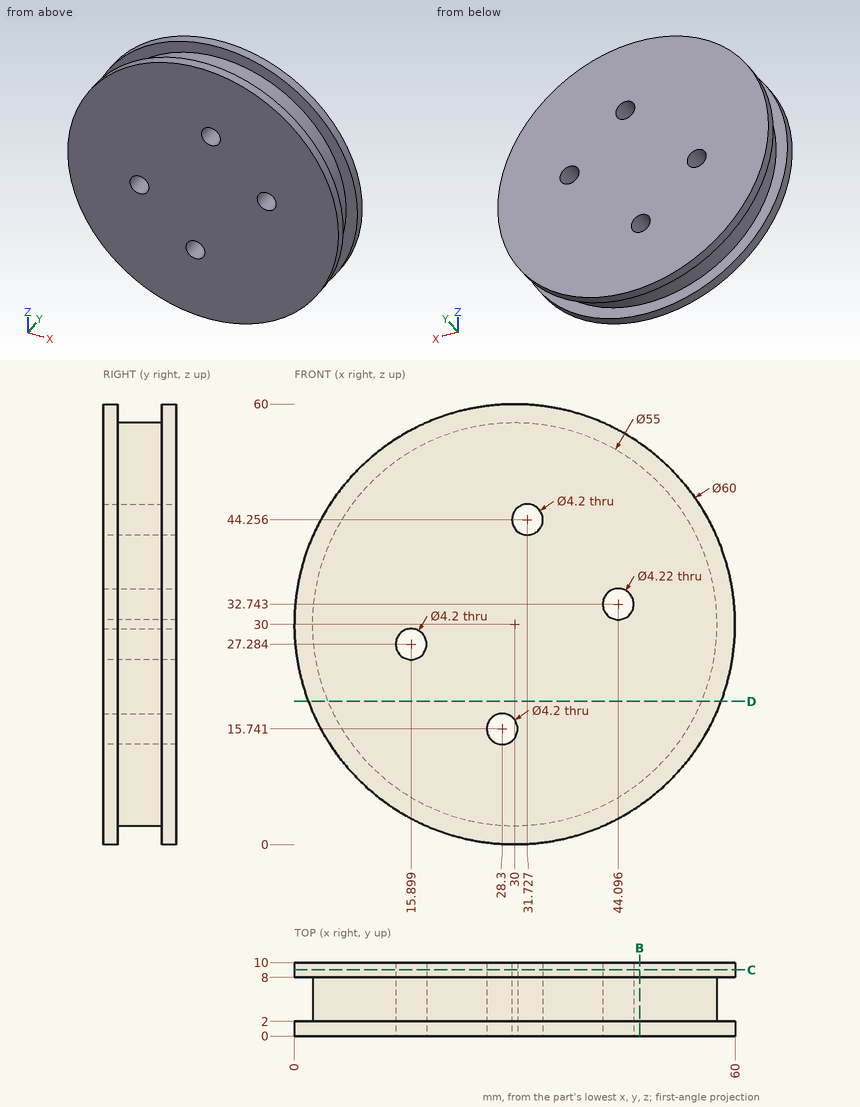
Input: dimensioned drawing with shaded views. Units: mm. Origin: part minimum x, y, z. Coordinates: 2 decimals unless noted, no trailing zeros. Write each loop counter-clockwise with the first axis right and the second up, starting at its lowest first coordinate (ties: lowest second). Pieces come first, ordered by that corner, then holes. Notation, with made-up numbers: M -26,-23 L 29,-23 A13 ccw 29,0 Z; hole C 34,-39.5 d10. An arc over 180 degrees is marked long. Answer as a JSON object with one key per item and string values. Group by question number.
(1) Section D-D on z = 19.5. Output: boundary loops of the cut face in (x, y), plus the area to 3 significant figures.
(2) Ray query, line 1 along Y through (x, z) = (58, 23); line 2 along Z through (x, y) = (32.5, 1.5) (1 decimal); line 3 along X through (y, z) = (5, 43) (1 decimal). Return the intervals inside material, ascending. Write a range as [from, to].
(3) Section B-B on x = 47. Output: boundary loops of the cut face in (y, z) (1 decimal).
(4) Contact query for a flat-ended pin moving along its axis: P1, Ø6, axis at x = 9.5, y = 4.5, coming from the -Z side (1 decimal). Output: stop coordinate, or through.
(5) Section C-C on y = 9. Output: boundary loops of the cut face in (x, z) (1 decimal), plus the area to 3 significant figures.
Result set:
{
 "1": {"outline": "M 1.9,0 L 58.1,0 L 58.1,2 L 55.42,2 L 55.42,8 L 58.1,8 L 58.1,10 L 1.9,10 L 1.9,8 L 4.58,8 L 4.58,2 L 1.9,2 Z", "area": "530 mm2"},
 "2": {"line 1": "y = [0, 2], [8, 10]", "line 2": "z = [0.1, 42.3], [46.2, 59.9]", "line 3": "x = [5.8, 30], [33.4, 54.2]"},
 "3": {"outline": "M 0,5.3 L 2,5.3 L 2,8.4 L 8,8.4 L 8,5.3 L 10,5.3 L 10,54.7 L 8,54.7 L 8,51.6 L 2,51.6 L 2,54.7 L 0,54.7 Z"},
 "4": {"P1": "stops at z = 6.7"},
 "5": {"outline": "C 30,30 d60; hole C 15.9,27.3 d4.2; hole C 28.3,15.7 d4.2; hole C 31.7,44.3 d4.2; hole C 44.1,32.7 d4.2", "area": "2,770 mm2"}
}
